The listing builds one solid part. Answer for the finished solid, in the listing's coordinates (mm). Round coordinates to 2 decimals unless told otherwise and drop trailing zeros. Return JSON: item names as keys, results as strings. Group by question number.
(1) Determine the mould class of faces 1 (the cylindrical face through (34.994, 0.011, 22.12)), 2 (the flat face through (-1, 0, 25)), 3 (the flat face through (-40, 0, 0)), 4 (the cylindrical face through (34.994, 0.011, -20.655)) for opening direction Z: +Z half, -Z half, draft (parallel to the pull), parting line (faces both ways), or undercut.
(2) Find the intervals of material crossed by line 1 along Z through (x, y) = (36.5, -0.45); line 2 along Z through (x, y) = (-35.5, 0.15); line 3 along X through (y, z) = (-0.7, 20.5), in increasing order. Write a range as [from, to].
(3) This flat-tipped pin is pushed along its axis until it touches: pin 1 (1.9 mm diameter, centred on x = 36.4, z = 21.39, fed in from -Y). Where does it stop, or does it pass through?
```python
from build123d import *

# Parameters (mm, degrees)
SKETCH1_W           = 80
SKETCH1_H           = 50
BOSS_EXTRUDE1_DEPTH = 0.8001
SKETCH2_R           = 1.5875
CUT_EXTRUDE1_DEPTH  = 48.197040586


with BuildPart() as part:
    # Sketch1 → Boss-Extrude1 (new, symmetric)
    with BuildSketch(Plane(origin=(0, 0, 0), x_dir=(1, 0, 0), z_dir=(0, 1, 0))):
        Rectangle(SKETCH1_W, SKETCH1_H)
    extrude(amount=BOSS_EXTRUDE1_DEPTH, both=True)

    # Sketch2 → Cut-Extrude1 (cut, through all)
    with BuildSketch(Plane(origin=(0, 0.8001, 0), x_dir=(1, 0, 0), z_dir=(0, 1, 0))):
        with Locations(Location((-36.40283621, 21.38740377, 0), (0, 0, 270))):
            Circle(SKETCH2_R)
        with Locations(Location((-36.40283621, -21.38740377, 0), (0, 0, 270))):
            Circle(SKETCH2_R)
        with Locations(Location((36.40283621, -21.38740377, 0), (0, 0, 270))):
            Circle(SKETCH2_R)
        with Locations(Location((36.40283621, 21.38740377, 0), (0, 0, 270))):
            Circle(SKETCH2_R)
    extrude(amount=-CUT_EXTRUDE1_DEPTH, mode=Mode.SUBTRACT)


solid = part.part
```
Working result:
{
 "1": {"face 1": "undercut", "face 2": "+Z half", "face 3": "draft", "face 4": "undercut"},
 "2": {"line 1": "z = [-25, -22.97], [-19.8, 19.8], [22.97, 25]", "line 2": "z = [-25, -22.69], [-20.08, 20.08], [22.69, 25]", "line 3": "x = [-40, -37.72], [-35.09, 35.09], [37.72, 40]"},
 "3": {"pin 1": "passes through"}
}
